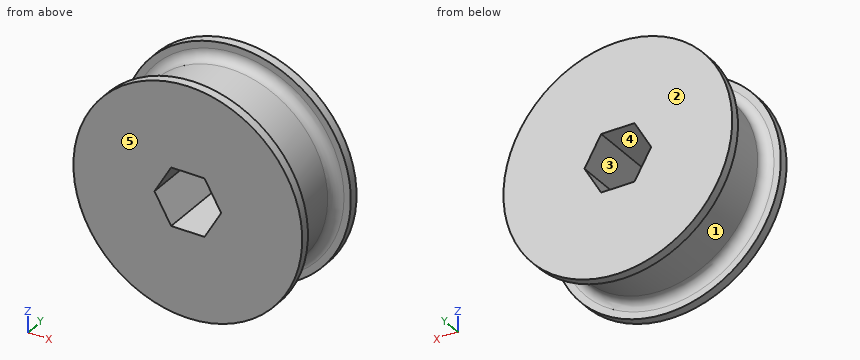
```python
from build123d import *

# Parameters (mm, degrees)
SKETCH1_R           = 25.4
SKETCH1_R_2         = 4.8387
BOSS_EXTRUDE1_DEPTH = 19.05
CUT_EXTRUDE1_DEPTH  = 41.659838908


with BuildPart() as part:
    # Sketch1 → Boss-Extrude1 (new body)
    with BuildSketch(Plane(origin=(0, 0, 0), x_dir=(1, 0, 0), z_dir=(0, 1, 0))):
        with Locations(Location((0, 0, 0), (0, 0, 90))):
            Circle(SKETCH1_R)
        with Locations(Location((0, 0, 0), (0, 0, 90))):
            Circle(SKETCH1_R_2, mode=Mode.SUBTRACT)
    extrude(amount=BOSS_EXTRUDE1_DEPTH)

    # Sketch6 → Cut-Extrude1 (cut, through all)
    with BuildSketch(Plane(origin=(0, 19.05, 0), x_dir=(1, 0, 0), z_dir=(0, 1, 0))):
        Polygon((3.702835951, -6.4135), (7.405671903, 0), (3.702835951, 6.4135), (-3.702835951, 6.4135), (-7.405671903, 0), (-3.702835951, -6.4135), align=None)
    extrude(amount=-CUT_EXTRUDE1_DEPTH, mode=Mode.SUBTRACT)

    # Sketch2 → Cut-Revolve1 (revolve, cut)
    with BuildSketch(Plane.XY, mode=Mode.PRIVATE) as cut_revolve1_sk:
        with BuildLine():
            Line((25.4, 17.04975), (23.876, 17.04975))
            ThreePointArc((23.876, 17.04975), (22.304455179, 16.398794821), (21.6535, 14.82725))
            Line((21.6535, 14.82725), (21.6535, 4.22275))
            ThreePointArc((21.6535, 4.22275), (22.304455179, 2.651205179), (23.876, 2.00025))
            Line((23.876, 2.00025), (25.4, 2.00025))
            Line((25.4, 2.00025), (25.4, 17.04975))
        make_face()
    revolve(cut_revolve1_sk.sketch.rotate(Axis((0, 0, 0), (0, 1, 0)), 90), axis=Axis((0, 0, 0), (0, 1, 0)), mode=Mode.SUBTRACT)


solid = part.part
```
Can you work these out from the model? Positions are in its coordinate system, mm. Face numbers are marked on the shaded views. A direction names the side the tool comes from. Give positions to 0.01 mm unless a question says otherwise; leave off trailing zeros. Loops run counter-clockwise (first coordinate to the right, second up) from the corner with the lowest first, then second, coordinate; pieces in that order, holes last. Notation, with made-up numbers: M 74,-10.75 L 124,-10.75 A20 ccw 124,10.25 Z; hole C 42.5,35 d9. An arc over 180 degrees is marked long. Use one line per item in the form item = value. Start each with the question number.
(1) On a 3-axis mill with a long thin cutter (end or side, diameter ignored), from which of +Z, -Z, +X, -X, +Y, -Y can I reach the whole of each face in a straight line? I mean the marked faces 4 and 5. Say none if no direction works.
(2) I want a section at C-C, the plane y = 16. Write out the boundary of the cut face in (x, z).
(3) Thinking about a two-plate mould opening in Z: for the marked faces 1, 2 and 3, which applies, released by +Z, released by -Z, zero draft, split by the parting line, or undercut?
(4) Please list where these lines run through material, in increasing order: line 1 (Y direction, x = -15, z = 20); line 2 (Z direction, x = 6, y = 17.75); line 3 (Z direction, x = -2, y = 4).
(5) I want a section at A-A, the plane y = 5.75. Write out the boundary of the cut face in (x, z), and give its area (3 significant figures).
(6) I'm going to push flat-ended pins straight in: P1, Ø8, axis at x = 19.5, y = 13.5, coming from the +Z side; P2, Ø1.5, axis at x = -2.5, y = 12.5, coming from the -Z side; P3, Ø5, axis at y = 8, z = 4.5, coming from the +X side. Where does each tip first touch, or does it pass through?
Worked out:
q1.face_4 = +Y, -Y
q1.face_5 = +Z, -Z, +X, -X, -Y
q2.outline = C 0,0 d43.98; hole M -7.41,0 L -3.7,-6.41 L 3.7,-6.41 L 7.41,0 L 3.7,6.41 L -3.7,6.41 Z
q3.face_1 = split by the parting line
q3.face_2 = zero draft
q3.face_3 = undercut
q4.line_1 = 0 to 2, 17.05 to 19.05
q4.line_2 = -24.68 to -2.43, 2.43 to 24.68
q4.line_3 = -21.57 to -6.41, 6.41 to 21.57
q5.outline = C 0,0 d43.31; hole M -7.41,0 L -3.7,-6.41 L 3.7,-6.41 L 7.41,0 L 3.7,6.41 L -3.7,6.41 Z
q5.area = 1,330 mm²
q6.P1 = 18.26
q6.P2 = -21.58
q6.P3 = 21.56
